from build123d import *

# Parameters (mm, degrees)
BOSS_EXTRUDE1_DEPTH     = 25.4
CUT_EXTRUDE2_REACH      = 47.575
CUT_EXTRUDE2_END_RADIUS = 49.2125
SKETCH4_R               = 1.27
CUT_EXTRUDE4_START      = -14.566377
SKETCH11_R              = 3.6576
CUT_EXTRUDE4_DEPTH      = 7.62
CUT_EXTRUDE5_REACH      = 67.474
CUT_EXTRUDE5_END_RADIUS = 49.2125
SKETCH15_R              = 1.8288
CHAMFER1_SIZE           = 2.54
CHAMFER1_SIZE2          = 5.08


with BuildPart() as part:
    # Sketch2 → Boss-Extrude1 (new body)
    with BuildSketch(Plane(origin=(0, 0, 0), x_dir=(1, 0, 0), z_dir=(0, 1, 0))):
        with BuildLine():
            Line((34.671523348, 34.925), (34.646123348, 34.925))
            Line((34.646123348, 34.925), (34.646123348, -34.925))
            Line((34.646123348, -34.925), (34.671523348, -34.925))
            ThreePointArc((34.671523348, -34.925), (49.2125, 0), (34.671523348, 34.925))
        make_face()
    extrude(amount=BOSS_EXTRUDE1_DEPTH)

    # Cut-Extrude2: up to this cylinder (the profile starts inside it)
    cut_extrude2_end = Plane(origin=(0, 12.7, 0), z_dir=(0, -1, 0)) * Cylinder(CUT_EXTRUDE2_END_RADIUS, 194.575, mode=Mode.PRIVATE)
    # Sketch4 → Cut-Extrude2 (cut, up to the surface)
    with BuildSketch(Plane.ZY.offset(-34.646123348), mode=Mode.PRIVATE) as cut_extrude2_sk1:
        with Locations((0, 12.7)):
            Circle(SKETCH4_R)
    cut_extrude2_tool1 = extrude(cut_extrude2_sk1.sketch, amount=-CUT_EXTRUDE2_REACH, mode=Mode.PRIVATE) & cut_extrude2_end
    add(cut_extrude2_tool1.solids().sort_by_distance((34.646123, 12.7, 0))[0], mode=Mode.SUBTRACT)

    # Sketch11 → Cut-Extrude4 (cut)
    with BuildSketch(Plane.ZY.offset(-34.646123348).offset(CUT_EXTRUDE4_START)):
        with Locations(Location((0, 12.7, 0), (0, 0, 180))):
            Circle(SKETCH11_R)
    extrude(amount=CUT_EXTRUDE4_DEPTH, mode=Mode.SUBTRACT)

    # Cut-Extrude5: up to this cylinder (the profile starts inside it)
    cut_extrude5_end = Plane(origin=(0, 12.7, 0), z_dir=(0, -1, 0)) * Cylinder(CUT_EXTRUDE5_END_RADIUS, 235.925334, mode=Mode.PRIVATE)
    # Sketch15 → Cut-Extrude5 (cut, up to the surface)
    with BuildSketch(Plane(origin=(0, 0, 0), x_dir=(0, 0, -1), z_dir=(1, 0, 0)), mode=Mode.PRIVATE) as cut_extrude5_sk1:
        with BuildLine():
            ThreePointArc((-18.9738, 12.7), (-17.145, 10.8712), (-15.3162, 12.7))
            Line((-15.3162, 12.7), (-18.9738, 12.7))
        make_face()
    cut_extrude5_tool1 = extrude(cut_extrude5_sk1.sketch, amount=CUT_EXTRUDE5_REACH, mode=Mode.PRIVATE) & cut_extrude5_end
    add(cut_extrude5_tool1.solids().sort_by_distance((0, 11.923833, 17.145))[0], mode=Mode.SUBTRACT)
    # Sketch15 → Cut-Extrude5 (cut, up to the surface)
    with BuildSketch(Plane(origin=(0, 0, 0), x_dir=(0, 0, -1), z_dir=(1, 0, 0)), mode=Mode.PRIVATE) as cut_extrude5_sk2:
        with BuildLine():
            Line((-18.9738, 12.7), (-15.3162, 12.7))
            ThreePointArc((-15.3162, 12.7), (-17.145, 14.5288), (-18.9738, 12.7))
        make_face()
    cut_extrude5_tool2 = extrude(cut_extrude5_sk2.sketch, amount=CUT_EXTRUDE5_REACH, mode=Mode.PRIVATE) & cut_extrude5_end
    add(cut_extrude5_tool2.solids().sort_by_distance((0, 13.476167, 17.145))[0], mode=Mode.SUBTRACT)
    # Sketch15 → Cut-Extrude5 (cut, up to the surface)
    with BuildSketch(Plane(origin=(0, 0, 0), x_dir=(0, 0, -1), z_dir=(1, 0, 0)), mode=Mode.PRIVATE) as cut_extrude5_sk3:
        with Locations(Location((17.145, 12.7, 0), (0, 0, 180))):
            Circle(SKETCH15_R)
    cut_extrude5_tool3 = extrude(cut_extrude5_sk3.sketch, amount=CUT_EXTRUDE5_REACH, mode=Mode.PRIVATE) & cut_extrude5_end
    add(cut_extrude5_tool3.solids().sort_by_distance((0, 12.7, -17.145))[0], mode=Mode.SUBTRACT)

    # Chamfer1
    chamfer1_edges = [part.edges().sort_by_distance(p)[0] for p in [
        (34.646123348, 0, 0),
    ]]
    chamfer1_side = [part.faces().sort_by_distance(p)[0] for p in [
        (40.553555626, 0, 0),
    ]]
    chamfer(chamfer1_edges, length=CHAMFER1_SIZE, length2=CHAMFER1_SIZE2, reference=chamfer1_side[0])


solid = part.part
Work out the finished part from the listing and answer in its coordinate system (mm). A direction names the side the tool comes from. Round coordinates to 2 decimals unless told otherwise and drop trailing zeros. Write each loop counter-clockwise with the first axis right and the second up, starting at its lowest first coordinate (ties: lowest second). Pieces come first, ordered by that corner, then holes. Notation, with made-up numbers: (13, 16) -> (71, 16) arc R23 ccw to (71, 49) -> close; hole circle Ø2 at (61.25, 52.25). An arc over 180 degrees is marked (long way). Answer as CSV lines item,"result". Start each with the question number.
(1) A tool of negligible diameter and unlimited length cuts with its end or side. For faces 1 (the cylindrical face through (45.46, 16.27, 0.79)), 2 (the flat face through (42, 0, 0)), from which of +Z, -Z, +X, -X, +Y, -Y can it reach the whole face along a straight path? Write none if from no direction.
(2) The part is cut by section A-A, the plane z = 0. Give the vertices of the cut face in (x, y).
(3) Find the intervals of material crossed by probe 1 along Y at (x, z) = (40.25, 0); probe 2 along Y at (x, z) = (43.5, 0); probe 3 along Z at (x, y) = (45, 12.7), in increasing order.
(4) The mould has two halves that part along Z. Classify faces 3 (the cylindrical face through (49.21, 6.88, 0.54)), 4 (the cylindrical face through (40.62, 12.15, -15.4)), 5 (the flat face through (35.898, 2.576, -0.489)): +Z half, -Z half, draft (parallel to the pull), parting line (faces both ways), or undercut.
(5) The part is cut by section B-B, the plane y = 12.7. Give the number of separate pieces and of enclosed holes in the cut face, then the cut area to 3 significant figures.
(6) Each of these flat-tipped pins is pushed along its axis until it touches: pin 1 (8 mm diameter, centred on x = 42, y = 7.5, fed in from -Z); pin 2 (5 mm diameter, centred on x = 41, y = 9.5, fed in from -Z); pin 3 (4 mm diameter, centred on x = 42, y = 18, fed in from +Z); pin 4 (8.5 mm diameter, centred on y = 12.7, z = 0, fed in from +X). Where does it stop, or does it pass through?
(7) The part is cut by section C-C, the plane x = 35.75. Give the vertices of the cut face in (y, z) (3 decimals), then the cut area to 3 significant figures.
Output values:
1,face 1,"+X"
1,face 2,"+Z, -Z, +X, -X, -Y"
2,outline,"(34.65, 5.08) -> (37.19, 0) -> (49.21, 0) -> (49.21, 9.04) -> (41.59, 9.04) -> (41.59, 11.43) -> (34.65, 11.43) -> close; (34.65, 13.97) -> (41.59, 13.97) -> (41.59, 16.36) -> (49.21, 16.36) -> (49.21, 25.4) -> (34.65, 25.4) -> close"
3,probe 1,"y = 0 to 11.43, 13.97 to 25.4"
3,probe 2,"y = 0 to 9.04, 16.36 to 25.4"
3,probe 3,"z = -19.92 to -18.97, -15.32 to -3.66, 3.66 to 15.32, 18.97 to 19.92"
4,face 3,"parting line"
4,face 4,"undercut"
4,face 5,"draft"
5,separate pieces,"4"
5,enclosed holes,"0"
5,area,"545 mm²"
6,pin 1,"stops at z = -31.27"
6,pin 2,"stops at z = -30.65"
6,pin 3,"stops at z = 28.67"
6,pin 4,"stops at x = 49.21"
7,outline,"(2.872, -33.82) -> (25.4, -33.82) -> (25.4, 33.82) -> (2.872, 33.82) -> close; hole circle Ø3.658 at (12.7, -17.145); hole circle Ø3.658 at (12.7, 17.145); hole circle Ø2.54 at (12.7, 0)"
7,area,"1,500 mm²"
